CAD build for the part. Positions are in the model's coordinates, mm. A direction names the side the tool comes from. Coordinates: 2 decimals unless noted, no trailing zeros. Loops run counter-clockwise (first coordinate to the right, second up) from the corner with the lowest first, then second, coordinate; pieces in that order, holes last.
1) Wall check: line 1 along X through (y, z) = (-87, 2.75); line 2 along Z through (x, y) = (35.5, -45); line 3 along Y through (x, z) = (12, 8.5). Give the ranges that are in metal, low to high.
2) Saw through at A-A, the plane z = 4. Give the number of separate pieces and of enclosed holes in the cut face, and give its area (3 significant figures).
3) Which spindle directions (+Z, -Z, +X, -X, +Y, -Y) get a long thin tool onto all of the face, cutting with end or side? Do faces 4 (the flat face through (56, -6, 7)), 5 (the flat face through (11, -98.45, 8)), 6 (the flat face through (50.5, -100, 5)), 7 (the cylindrical face through (56.867, -76.384, 4.465)). Say none if no direction does.
4) Two-plate mould, pull along X, no slides. Class faces 1 (the flat face through (31, -51, 0)), 2 (the flat face through (0, -52, 1)), 3 (the flat face through (9, -100, 4)): +X half, -X half, draft (parallel to the pull), parting line (faces both ways), or undercut.
5) Saw through at C-C, the plane x = 16.5. Write the cut outline in (y, z).
6) Pin check, flat tips, straight feed: pin 1 Ø3 at (x, y) = (26.5, -91) entering from +Z; pin 2 Ø4 at (x, y) = (46.5, -58) entering from +Z; pin 3 Ø2 at (y, z) = (-89.5, 5) entering from -X; pin 4 Ø1 at (y, z) = (-19, 4) entering from -X. Stop position of each tip, or through.
7) Saw through at B-B, the plane y = -6.45. Write the cut outline in (x, z).
8) Saw through at D-D, the plane y = -39.5. Write the cut outline in (x, z), and give its area (3 significant figures).
```python
from build123d import *

# Parameters (mm, degrees)
P_IDAT_VYSUNUT_M1_DEPTH   = 2
SKICA3_R                  = 2.45
P_IDAT_VYSUNUT_M3_DEPTH   = 5
P_IDAT_VYSUNUT_M4_DEPTH   = 37.5
SKICA8_W                  = 10
SKICA8_H                  = 10
ODEBRAT_VYSUNUT_M2_DEPTH  = 136.974087605
SKICA10_W                 = 27.5
SKICA10_H                 = 79
ODEBRAT_VYSUNUT_M3_DEPTH  = 3
P_IDAT_VYSUNUT_M5_DEPTH   = 1
SKICA13_W                 = 3
SKICA13_H                 = 36.5
ODEBRAT_VYSUNUT_M6_DEPTH  = 127.590886323
SKICA14_W                 = 3
SKICA14_H                 = 36.5
ODEBRAT_VYSUNUT_M7_DEPTH  = 127.590886323
SKICA15_W                 = 36.5
SKICA15_H                 = 3
ODEBRAT_VYSUNUT_M8_DEPTH  = 136.974087605
SKICA19_W                 = 37
SKICA19_H                 = 13
ODEBRAT_VYSUNUT_M9_DEPTH  = 132.581543159
SKICA20_W                 = 63
SKICA20_H                 = 102.45
SKICA20_W_2               = 57
SKICA20_H_2               = 79
ODEBRAT_VYSUNUT_M10_DEPTH = 1
SKICA22_W                 = 8
SKICA22_H                 = 4
SKICA22_W_2               = 6
SKICA22_H_2               = 5
P_IDAT_VYSUNUT_M6_DEPTH   = 7
SKICA23_W                 = 4
SKICA23_H                 = 5
SKICA23_W_2               = 2
ODEBRAT_VYSUNUT_M12_DEPTH = 5
SKICA25_W                 = 4
SKICA25_H                 = 16
SKICA25_W_2               = 1
SKICA25_H_2               = 13
P_IDAT_VYSUNUT_M8_DEPTH   = 6.5


with BuildPart() as part:
    # Skica1 → Přidat vysunutím1 (new body)
    with BuildSketch(Plane.XY):
        Polygon((13, -102.45), (13, -115.45), (50, -115.45), (50, -102.45), (63, -102.45), (63, 0), (0, 0), (0, -102.45), align=None)
    extrude(amount=P_IDAT_VYSUNUT_M1_DEPTH)

    # Skica3 → Přidat vysunutím3 (add)
    with BuildSketch(Plane.XY.offset(2)):
        with Locations((7.55, -6.45)):
            Circle(SKICA3_R)
        with Locations((7.55, -78.45)):
            Circle(SKICA3_R)
        with Locations((55.55, -78.45)):
            Circle(SKICA3_R)
        with Locations((55.55, -6.45)):
            Circle(SKICA3_R)
    extrude(amount=P_IDAT_VYSUNUT_M3_DEPTH)

    # Skica4 → Přidat vysunutím4 (add)
    with BuildSketch(Plane.XY.offset(2)):
        Polygon((63, 0), (63, -102.45), (60, -102.45), (60, -3), (3, -3), (3, -102.45), (0, -102.45), (0, 0), align=None)
    extrude(amount=P_IDAT_VYSUNUT_M4_DEPTH)

    # Skica8 → Odebrat vysunutím2 (cut, through all)
    with BuildSketch(Plane.ZY.offset(-60)):
        with Locations((7, -49)):
            Rectangle(SKICA8_W, SKICA8_H)
    extrude(amount=-ODEBRAT_VYSUNUT_M2_DEPTH, mode=Mode.SUBTRACT)

    # Skica10 → Odebrat vysunutím3 (cut)
    with BuildSketch(Plane.ZY):
        with Locations((25.75, -42.5)):
            Rectangle(SKICA10_W, SKICA10_H)
    extrude(amount=-ODEBRAT_VYSUNUT_M3_DEPTH, mode=Mode.SUBTRACT)

    # Skica11 → Přidat vysunutím5 (add)
    with BuildSketch(Plane.XY.offset(2)):
        Polygon((3, -82), (60, -82), (60, -102.45), (50, -102.45), (50, -115.45), (13, -115.45), (13, -102.45), (3, -102.45), align=None)
    extrude(amount=P_IDAT_VYSUNUT_M5_DEPTH)

    # Skica13 → Odebrat vysunutím6 (cut, through all)
    with BuildSketch(Plane.XZ.offset(102.45)):
        with Locations((1.5, 21.25)):
            Rectangle(SKICA13_W, SKICA13_H)
    extrude(amount=-ODEBRAT_VYSUNUT_M6_DEPTH, mode=Mode.SUBTRACT)

    # Skica14 → Odebrat vysunutím7 (cut, through all)
    with BuildSketch(Plane.XZ.offset(102.45)):
        with Locations((61.5, 21.25)):
            Rectangle(SKICA14_W, SKICA14_H)
    extrude(amount=-ODEBRAT_VYSUNUT_M7_DEPTH, mode=Mode.SUBTRACT)

    # Skica15 → Odebrat vysunutím8 (cut, through all)
    with BuildSketch(Plane.ZY.offset(-3)):
        with Locations((21.25, -1.5)):
            Rectangle(SKICA15_W, SKICA15_H)
    extrude(amount=-ODEBRAT_VYSUNUT_M8_DEPTH, mode=Mode.SUBTRACT)

    # Skica19 → Odebrat vysunutím9 (cut, through all)
    with BuildSketch(Plane.XY.offset(3)):
        with Locations((31.5, -108.95)):
            Rectangle(SKICA19_W, SKICA19_H)
    extrude(amount=-ODEBRAT_VYSUNUT_M9_DEPTH, mode=Mode.SUBTRACT)

    # Skica20 → Odebrat vysunutím10 (cut)
    with BuildSketch(Plane.XY.offset(3)):
        with Locations((31.5, -51.225)):
            Rectangle(SKICA20_W, SKICA20_H)
        with Locations((31.5, -42.5)):
            Rectangle(SKICA20_W_2, SKICA20_H_2, mode=Mode.SUBTRACT)
    extrude(amount=-ODEBRAT_VYSUNUT_M10_DEPTH, mode=Mode.SUBTRACT)

    # Skica22 → Přidat vysunutím6 (add)
    with BuildSketch(Plane.XY.offset(2)):
        with Locations((11, -100.45)):
            Rectangle(SKICA22_W, SKICA22_H)
        with Locations((53.5, -99.95)):
            Rectangle(SKICA22_W_2, SKICA22_H_2)
    extrude(amount=P_IDAT_VYSUNUT_M6_DEPTH)

    # Skica23 → Odebrat vysunutím12 (cut)
    with BuildSketch(Plane.XZ.offset(102.45)):
        with Locations((11, 4.5)):
            Rectangle(SKICA23_W, SKICA23_H)
        with Locations((53.5, 4.5)):
            Rectangle(SKICA23_W_2, SKICA23_H)
    extrude(amount=-ODEBRAT_VYSUNUT_M12_DEPTH, mode=Mode.SUBTRACT)

    # Skica25 → Přidat vysunutím8 (add)
    with BuildSketch(Plane.XY.offset(2)):
        with Locations((26, -92.45)):
            Rectangle(SKICA25_W, SKICA25_H)
        with Locations((26, -92.45)):
            Rectangle(SKICA25_W_2, SKICA25_H_2, mode=Mode.SUBTRACT)
    extrude(amount=P_IDAT_VYSUNUT_M8_DEPTH)


solid = part.part
```
Data:
1. line 1: x = 24 to 25.5, 26.5 to 28
1. line 2: z = 0 to 2
1. line 3: y = -102.45 to -98.45
2. separate pieces: 9
2. enclosed holes: 1
2. area: 162 mm2
3. face 4: +Z, +X, -X, +Y
3. face 5: +Z, -X
3. face 6: +Z, +Y, -Y
3. face 7: +Z
4. face 1: draft
4. face 2: -X half
4. face 3: undercut
5. outline: (-102.45, 0) - (0, 0) - (0, 2) - (-102.45, 2) - close
6. pin 1: stops at z = 8.5
6. pin 2: stops at z = 2
6. pin 3: stops at x = 24
6. pin 4: passes through
7. outline: (0, 0) - (63, 0) - (63, 2) - (58, 2) - (58, 7) - (53.1, 7) - (53.1, 2) - (10, 2) - (10, 7) - (5.1, 7) - (5.1, 2) - (0, 2) - close
8. outline: (0, 0) - (63, 0) - (63, 2) - (0, 2) - close
8. area: 126 mm2
